```python
from build123d import *

# Parameters (mm, degrees)
F1_DEPTH = 12.7
F2_R     = 3.175
F3_DEPTH = 41.5002601562
F4_W     = 130.419023335
F4_H     = 4.1049833633
F5_DEPTH = 25
F6_R     = 2
F7_R     = 0.432
F9_DEPTH = 12.7
F10_R    = 1


# Not quite as in the source:
# - ends of sketch curves that miss each other by under 0.0002 mm in the source are joined
# - the dataset's text gives a spline's control points without its knots; the knots are read off the source's solid


with BuildPart() as f1:
    # F0 (on Front) → F1 (new body)
    with BuildSketch(Plane.XZ):
        with BuildLine():
            Line((-8, 0), (0, 0))
            add(Edge.make_bspline(
                [(0, 0), (0, 16.0348825157), (7.430841215, 33.6514413357), (23.5, 33.5)],
                knots=[0, 0, 0, 0, 40.9206549312, 40.9206549312, 40.9206549312, 40.9206549312], degree=3))
            add(Edge.make_bspline(
                [(47, 0), (47, 16.0348825157), (39.569158785, 33.6514413357), (23.5, 33.5)],
                knots=[0, 0, 0, 0, 40.9206549312, 40.9206549312, 40.9206549312, 40.9206549312], degree=3))
            Line((47, 0), (55, 0))
            add(Edge.make_bspline(
                [(55, 0), (55, 2.3133051501), (54.8084752548, 5.6604865088), (54.3346414744, 8.9941225704), (54.1644875118, 10.0000161913)],
                knots=[0, 0, 0, 0, 0.125, 0.1792883855, 0.1792883855, 0.1792883855, 0.1792883855], degree=3))
            add(Edge.make_bspline(
                [(54.1644875118, 10.0000161913), (53.9428588652, 11.3102110198), (53.2041802455, 14.9199242801), (51.403557473, 20.6965522199), (48.312647429, 27.0635606249), (44.7757382973, 31.8590791464), (41.27501086, 35.2044913237), (38.3020149436, 37.39930019), (34.9881581098, 39.2038242784), (31.3670929719, 40.5407901401), (27.6491274865, 41.3170292606), (25.11417344, 41.4919330376), (23.9092731988, 41.5002601562)],
                knots=[0.1792883855, 0.1792883855, 0.1792883855, 0.1792883855, 0.25, 0.375, 0.5, 0.625, 0.6875, 0.75, 0.8125, 0.875, 0.9375, 0.9926226885, 0.9926226885, 0.9926226885, 0.9926226885], degree=3))
            Line((23.9092731988, 41.5002601562), (23.5, 41.5002601562))
            Line((23.5, 41.5002601562), (23.0907268012, 41.5002601562))
            add(Edge.make_bspline(
                [(-7.1644875118, 10.0000161913), (-6.9428588652, 11.3102110198), (-6.2041802455, 14.9199242801), (-4.403557473, 20.6965522199), (-1.312647429, 27.0635606249), (2.2242617027, 31.8590791464), (5.72498914, 35.2044913237), (8.6979850564, 37.39930019), (12.0118418902, 39.2038242784), (15.6329070281, 40.5407901401), (19.3508725135, 41.3170292606), (21.88582656, 41.4919330376), (23.0907268012, 41.5002601562)],
                knots=[0.1792883855, 0.1792883855, 0.1792883855, 0.1792883855, 0.25, 0.375, 0.5, 0.625, 0.6875, 0.75, 0.8125, 0.875, 0.9375, 0.9926226885, 0.9926226885, 0.9926226885, 0.9926226885], degree=3))
            add(Edge.make_bspline(
                [(-8, 0), (-8, 2.3133051501), (-7.8084752548, 5.6604865088), (-7.3346414744, 8.9941225704), (-7.1644875118, 10.0000161913)],
                knots=[0, 0, 0, 0, 0.125, 0.1792883855, 0.1792883855, 0.1792883855, 0.1792883855], degree=3))
        make_face()
        with BuildLine():
            Line((-35, 0), (-8, 0))
            add(Edge.make_bspline(
                [(-8, 0), (-8, 2.3133051501), (-7.8084752548, 5.6604865088), (-7.3346414744, 8.9941225704), (-7.1644875118, 10.0000161913)],
                knots=[0, 0, 0, 0, 0.125, 0.1792883855, 0.1792883855, 0.1792883855, 0.1792883855], degree=3))
            Line((-7.1644875118, 10.0000161913), (-35, 10))
            Line((-35, 10), (-35, 0))
        make_face()
        with BuildLine():
            Line((-35, 10), (-7.1643917939, 10))
            add(Edge.make_bspline(
                [(-7.1643917939, 10), (-6.9428588652, 11.3102110198), (-6.2041802455, 14.9199242801), (-4.403557473, 20.6965522199), (-1.312647429, 27.0635606249), (2.2242617027, 31.8590791464), (5.72498914, 35.2044913237), (8.6979850564, 37.39930019), (12.0118418902, 39.2038242784), (15.6329070281, 40.5407901401), (19.3508725135, 41.3170292606), (21.88582656, 41.4919330376), (23.0907268012, 41.5002601562)],
                knots=[0.1792883855, 0.1792883855, 0.1792883855, 0.1792883855, 0.25, 0.375, 0.5, 0.625, 0.6875, 0.75, 0.8125, 0.875, 0.9375, 0.9926226885, 0.9926226885, 0.9926226885, 0.9926226885], degree=3))
            Line((23.0907268012, 41.5002601562), (-12, 41.5002601562))
            Line((-12, 41.5002601562), (-12, 38.0002601562))
            Line((-12, 38.0002601562), (-15, 38.0002601562))
            Line((-15, 38.0002601562), (-18, 38.0002601562))
            Line((-18, 38.0002601562), (-18, 41.5002601562))
            Line((-18, 41.5002601562), (-35, 41.5002601562))
            Line((-35, 41.5002601562), (-35, 10))
        make_face()
        with BuildLine():
            add(Edge.make_bspline(
                [(55, 0), (55, 2.3133051501), (54.8084752548, 5.6604865088), (54.3346414744, 8.9941225704), (54.1644875118, 10.0000161913)],
                knots=[0, 0, 0, 0, 0.125, 0.1792883855, 0.1792883855, 0.1792883855, 0.1792883855], degree=3))
            Line((55, 0), (82, 0))
            Line((82, 0), (82, 10))
            Line((82, 10), (54.1644875118, 10.0000161913))
        make_face()
        with BuildLine():
            add(Edge.make_bspline(
                [(23.0907268012, 41.5002601562), (23.2269381476, 41.5012015188), (23.3633657228, 41.5012017791), (23.499999998, 41.5002598872)],
                knots=[0.9926226885, 0.9926226885, 0.9926226885, 0.9926226885, 0.9988541884, 0.9988541884, 0.9988541884, 0.9988541884], degree=3))
            Line((23.0907268012, 41.5002601562), (23.499999998, 41.5002598872))
        make_face()
        with BuildLine():
            add(Edge.make_bspline(
                [(54.1644875118, 10.0000161913), (53.9428588652, 11.3102110198), (53.2041802455, 14.9199242801), (51.403557473, 20.6965522199), (48.312647429, 27.0635606249), (44.7757382973, 31.8590791464), (41.27501086, 35.2044913237), (38.3020149436, 37.39930019), (34.9881581098, 39.2038242784), (31.3670929719, 40.5407901401), (27.6491274865, 41.3170292606), (25.11417344, 41.4919330376), (23.9092731988, 41.5002601562)],
                knots=[0.1792883855, 0.1792883855, 0.1792883855, 0.1792883855, 0.25, 0.375, 0.5, 0.625, 0.6875, 0.75, 0.8125, 0.875, 0.9375, 0.9926226885, 0.9926226885, 0.9926226885, 0.9926226885], degree=3))
            Line((54.1644875118, 10.0000161913), (82, 10))
            Line((82, 10), (82, 41.5002601562))
            Line((82, 41.5002601562), (23.9092731988, 41.5002601562))
        make_face()
        with BuildLine():
            add(Edge.make_bspline(
                [(23.9092731988, 41.5002601562), (23.7730618524, 41.5012015188), (23.6366342772, 41.5012017791), (23.500000002, 41.5002598872)],
                knots=[0.9926226885, 0.9926226885, 0.9926226885, 0.9926226885, 0.9988541884, 0.9988541884, 0.9988541884, 0.9988541884], degree=3))
            Line((23.500000002, 41.5002598872), (23.9092731988, 41.5002601562))
        make_face()
        Polygon((-12, 38.0002601562), (-12, 41.5002601562), (-15, 41.5002601562), (-18, 41.5002601562), (-18, 38.0002601562), (-15, 38.0002601562), align=None)
    extrude(amount=F1_DEPTH)

    # F2 (on face) → F3 (cut, through all)
    with BuildSketch(Plane.XY.offset(41.5002601562)):
        with Locations((-26.999999998, -6.35)):
            Circle(F2_R)
        with Locations((74.000000002, -6.35)):
            Circle(F2_R)
    extrude(amount=-F3_DEPTH, mode=Mode.SUBTRACT)

    # F4 (on Front) → F5 (cut)
    with BuildSketch(Plane.XZ):
        with Locations((22.7671675384, -1.0524916817)):
            Rectangle(F4_W, F4_H)
    extrude(amount=F5_DEPTH, mode=Mode.SUBTRACT)

    # F6
    f6_edges = [f1.edges().sort_by_distance(p)[0] for p in [
        (82, -6.35, 41.50026),
        (-35, -6.35, 41.50026),
    ]]
    fillet(f6_edges, radius=F6_R)

    # F7
    f7_edges = [f1.edges().sort_by_distance(p)[0] for p in [
        (-35, -6.35, 1),
        (0.009608, -6.35, 1),
        (46.990392, -6.35, 1),
        (82, -6.35, 1),
    ]]
    fillet(f7_edges, radius=F7_R)

    # F8 (on face) → F9 (cut, through all)
    with BuildSketch(Plane.XZ.offset(12.7)):
        Polygon((-18, 35.0002601562), (-12, 35.0002601562), (-6, 35.0002601562), (-6, 41.5002601562), (-12, 41.5002601562), (-18, 41.5002601562), align=None)
        Polygon((59.0000000039, 35.0002601562), (65.0000000039, 35.0002601562), (65.0000000039, 41.5002601562), (59.0000000039, 41.5002601562), (53.0000000039, 41.5002601562), (53.0000000039, 35.0002601562), align=None)
    extrude(amount=-F9_DEPTH, mode=Mode.SUBTRACT)

    # F10
    f10_edges = [f1.edges().sort_by_distance(p)[0] for p in [
        (-18, -6.35, 35.00026),
        (-6, -6.35, 35.00026),
        (-18, -6.35, 41.50026),
        (-6, -6.35, 41.50026),
        (53, -6.35, 35.00026),
        (53, -6.35, 41.50026),
        (65, -6.35, 35.00026),
        (65, -6.35, 41.50026),
    ]]
    fillet(f10_edges, radius=F10_R)


solid = f1.part
```
Model file for the job. Use its own axes, mm. A direction names the side the tool comes from. Coordinates: 2 decimals unless noted, no trailing zeros. Order: outer loops, then holes, each group sorted by start corner. A loop starts at its lowest first (then second) coordinate and runs counter-clockwise, first axis right, second up. Notation, with made-up numbers: (1, -16.5) - (45, -16.5) arc R26 cw to (45, 3.5) - close; hole circle Ø10 at (41.25, -12.5). An arc over 180 degrees is marked (long way). Return JSON: item names as keys, results as strings. Group by question number.
1) Tool access for faces 1 (the flat face through (-18, -6, 38)), 2 (the flat face through (38, -6, 41.5)): list every direction of +Z, -Z, +X, -X, +Y, -Y with a clear straight run to the whole face (end or side of a thin tool).
2) Flat gauge pin, fed straight in: P1, Ø5, axis at x = 74, y = -6.35, coming from the +Z side. Where does the tip first touch, or does it go through?
3) Saw through at D-D, the plane x = -14.5. Write the cut outline in (y, z), plus the area to 3 significant figures.
4) Saw through at A-A, the plane x = -27. Write the cut outline in (y, z) (3 decimals).
5) Probe line 1 (Y direction, x = 74, z = 27) (3 decimals); line 2 (X direction, y = -8.25, z = 3); line 3 (X direction, y = -4.25, z = 5). List the from-to ranges inside material, lowest first. Write a range as from..to.
6) Mould opens along Y. For faces 3 (the flat face through (23, -12.7, 35)), 4 (the cylindrical face through (77.03, -5.4, 21.53)), 5 (the flat face through (-23, -6, 41.5)) say: released by +Y, released by -Y, zero draft, split by the parting line, or undercut.
7) Saw through at B-B, the plane y = -6.35. Count the separate pieces of the cut face and the enclosed holes in it, plus the area to 3 significant figures.
Values found:
{
 "1": {"face 1": "+Z, +Y, -Y", "face 2": "+Z, +X, -X, +Y, -Y"},
 "2": {"P1": "passes through"},
 "3": {"outline": "(-12.7, 1) - (0, 1) - (0, 35) - (-12.7, 35) - close", "area": "432 mm²"},
 "4": {"outline": "(-12.7, 1) - (-9.525, 1) - (-9.525, 41.5) - (-12.7, 41.5) - close; (-3.175, 1) - (0, 1) - (0, 41.5) - (-3.175, 41.5) - close"},
 "5": {"line 1": "y = -12.7..-9.525, -3.175..0", "line 2": "x = -35..-29.54, -24.46..0.09, 46.91..71.46, 76.54..82", "line 3": "x = -35..-29.38, -24.62..0.24, 46.76..71.62, 76.38..82"},
 "6": {"face 3": "released by -Y", "face 4": "undercut", "face 5": "zero draft"},
 "7": {"separate pieces": "3", "enclosed holes": "0", "area": "2,850 mm²"}
}
